Part model, mm, in its own coordinate system. Face numbers are marked on the shaded views. A direction names the side the tool comes from. Coordinates: 2 decimals unless noted, no trailing zeros. Order: outer loops, then holes, each group sorted by start corner. A loop starts at its lowest first (then second) coordinate and runs counter-clockwise, first axis right, second up.
from build123d import *

# Parameters (mm, degrees)
SKETCH3_R               = 3.429
CUT_EXTRUDE1_DEPTH      = 1
CUT_EXTRUDE1_DEPTH_BACK = 11.922
CHAMFER1_SIZE           = 1.016


with BuildPart() as part:
    # Sketch2 → Revolve1 (revolve)
    with BuildSketch(Plane.XY):
        Polygon((10.922, 0), (0, 0), (0, 8.001), (2.032, 8.001), (2.032, 3.937), (6.858, 3.937), (6.858, 8.001), (10.922, 8.001), align=None)
    revolve(axis=Axis((10.922, 0, 0), (-1, 0, 0)))

    # Sketch3 → Cut-Extrude1 (cut, two sides)
    with BuildSketch(Plane(origin=(10.922, 0, 0), x_dir=(0, 0, -1), z_dir=(1, 0, 0))) as cut_extrude1_sk:
        Circle(SKETCH3_R)
    extrude(amount=CUT_EXTRUDE1_DEPTH, mode=Mode.SUBTRACT)
    extrude(cut_extrude1_sk.sketch, amount=-CUT_EXTRUDE1_DEPTH_BACK, mode=Mode.SUBTRACT)

    # Chamfer1
    chamfer1_edges = [part.edges().sort_by_distance(p)[0] for p in [
        (10.922, 0, 3.429),
    ]]
    chamfer(chamfer1_edges, length=CHAMFER1_SIZE)


solid = part.part
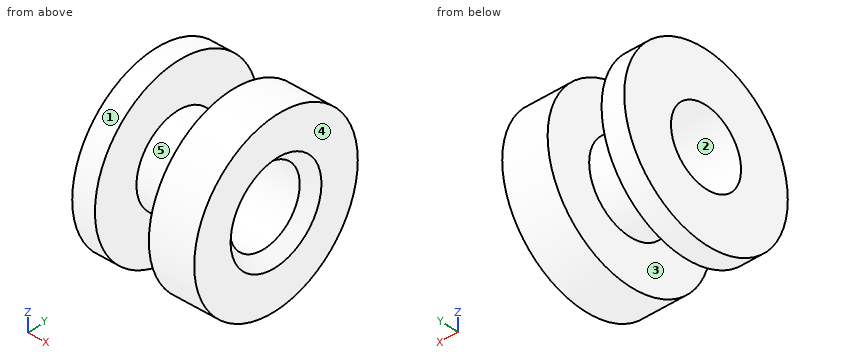
Q1. Mould opens along Y. For the marked faces 1, 2 and 3 say: pulls with the +Y half, pulls with the -Y half, needs draft (parallel to the pull), parting line crosses it, or undercut.
Results list:
face 1: parting line crosses it
face 2: undercut
face 3: needs draft
Q2. Pin check, flat tips, straight feed: pin 1 Ø4 at (y, z) = (0, 0.5) entering from +X; pin 2 Ø4 at (x, z) = (2.5, 4) entering from -Y; pin 3 Ø8 at (y, z) = (0, 0) entering from +X; pin 4 Ø3 at (x, z) = (4, -5) entering from -Y. Stop position of each tip, or through.
Results list:
pin 1: passes through
pin 2: stops at y = -7.73
pin 3: stops at x = 10.48
pin 4: stops at y = -1.8
Q3. Cut at C-C on x = 5.25. Write the cut outline in (y, z), and give its area (3 significant figures).
Results list:
outline: circle Ø7.87 at (0, 0); hole circle Ø6.86 at (0, 0)
area: 11.8 mm2
Q4. Cut at A-A on y = 0. Write the cut outline in (x, z) (3 decimals).
Results list:
outline: (0, -8.001) - (2.032, -8.001) - (2.032, -3.937) - (6.858, -3.937) - (6.858, -8.001) - (10.922, -8.001) - (10.922, -4.445) - (9.906, -3.429) - (0, -3.429) - close; (0, 3.429) - (9.906, 3.429) - (10.922, 4.445) - (10.922, 8.001) - (6.858, 8.001) - (6.858, 3.937) - (2.032, 3.937) - (2.032, 8.001) - (0, 8.001) - close
Q5. Which spindle directions (+Z, -Z, +X, -X, +Y, -Y) get a long thin tool onto all of the face, cutting with end or side? Do the marked faces 4 and 5. Say none if no direction does.
Results list:
face 4: +Z, -Z, +X, +Y, -Y
face 5: none
Q6. Wall check: line 1 along Y through (x, z) = (6, 0); line 2 along X through (y, z) = (-4.25, 3.75); line 3 along Z through (x, y) = (5.75, -0.5). Give the ranges that are in metal, low to high.
Results list:
line 1: y = -3.94 to -3.43, 3.43 to 3.94
line 2: x = 0 to 2.03, 6.86 to 10.92
line 3: z = -3.91 to -3.39, 3.39 to 3.91
Q7. Cut at D-D on y = -6.5. Write the cut outline in (x, z).
Results list:
outline: (0, -4.67) - (2.03, -4.67) - (2.03, 4.67) - (0, 4.67) - close; (6.86, -4.67) - (10.92, -4.67) - (10.92, 4.67) - (6.86, 4.67) - close
